The model under review builds one solid part; all positions refer to its coordinate system, in mm. Round coordinates to 2 decimals unless told otherwise and drop trailing zeros. Order: outer loops, then holes, each group sorted by start corner. A loop starts at its lowest first (then second) coordinate and runs counter-clockwise, first axis right, second up.
1) Consider section D-D (x = -16). Give the boundary of the cut face in (y, z).
2) Consider section C-C (y = -1.05). Give the number of separate pieces and of enclosed holes in the cut face, then the cut area to 3 significant figures.
3) Consider section A-A (x = 4). Give the boundary of the cut face in (y, z).
4) To check wall thickness, follow L1, parallel to Z at x = -4, y = 0.75; L2, parallel to X at y = 0.7, z = 35; L3, parallel to X at y = -0.25, z = 54.5. State the ranges of each line that lie inside material, in increasing order.
5) Consider section B-B (z = -15). Give the boundary of the cut face in (x, y), then the cut area to 3 significant figures.
from build123d import *

# Parameters (mm, degrees)
SKETCH1_W            = 50
SKETCH1_H            = 80
SKETCH1_W_2          = 23
SKETCH1_H_2          = 17
BOSS_EXTRUDE1_DEPTH  = 1.5875
M2_CLEARANCE_HOLE1_D = 2.4
M4_CLEARANCE_HOLE1_D = 4.5


with BuildPart() as part:
    # Sketch1 → Boss-Extrude1 (new, symmetric)
    with BuildSketch(Plane(origin=(0, 0, 0), x_dir=(1, 0, 0), z_dir=(0, 1, 0))):
        Polygon((-25, -40), (-11.5, -57), (-11.5, -40), align=None)
        Polygon((11.5, -40), (11.5, -57), (25, -40), align=None)
        Rectangle(SKETCH1_W, SKETCH1_H)
        with Locations((0, -48.5)):
            Rectangle(SKETCH1_W_2, SKETCH1_H_2)
    extrude(amount=BOSS_EXTRUDE1_DEPTH, both=True)

    # M2 Clearance Hole1 (through all)
    with Locations(Plane(origin=(0, 1.5875, 0), x_dir=(1, 0, 0), z_dir=(0, 1, 0))):
        with Locations((-4, -54.5), (4, -54.5), (4, -42.5), (-4, -42.5)):
            Hole(M2_CLEARANCE_HOLE1_D / 2)

    # M4 Clearance Hole1 (through all)
    with Locations(Plane(origin=(0, 1.5875, 0), x_dir=(1, 0, 0), z_dir=(0, 1, 0))):
        with Locations((-20, 15), (20, 15), (20, -35), (-20, -35)):
            Hole(M4_CLEARANCE_HOLE1_D / 2)


solid = part.part
Answer below:
1. outline: (-1.59, -40) - (1.59, -40) - (1.59, 51.33) - (-1.59, 51.33) - close
2. separate pieces: 1
2. enclosed holes: 8
2. area: 4,540 mm2
3. outline: (-1.59, -40) - (1.59, -40) - (1.59, 41.3) - (-1.59, 41.3) - close; (-1.59, 43.7) - (1.59, 43.7) - (1.59, 53.3) - (-1.59, 53.3) - close; (-1.59, 55.7) - (1.59, 55.7) - (1.59, 57) - (-1.59, 57) - close
4. L1: z = -40 to 41.3, 43.7 to 53.3, 55.7 to 57
4. L2: x = -25 to -22.25, -17.75 to 17.75, 22.25 to 25
4. L3: x = -13.49 to -5.2, -2.8 to 2.8, 5.2 to 13.49
5. outline: (-25, -1.59) - (-22.25, -1.59) - (-22.25, 1.59) - (-25, 1.59) - close; (-17.75, -1.59) - (17.75, -1.59) - (17.75, 1.59) - (-17.75, 1.59) - close; (22.25, -1.59) - (25, -1.59) - (25, 1.59) - (22.25, 1.59) - close
5. area: 130 mm2
